Could you check a few things on this drawing? It's one solid part, dimensions in mm from its lowest x, y, z. Give positions to 0.01 mm unless a question says otherwise; leave off trailing zeros. Loops run counter-clockwise (first coordinate to the right, second up) from the corner with the lowest first, then second, coordinate; pieces in that order, holes last. Notation, with made-up numbers: M 32,-20 L 52,-20 A17 ccw 52,-2 Z; hole C 9.25,89 d2. An arc over 180 degrees is marked long. Answer as CSV lines item,"result". Start each with the question number.
Item 1: I want a section at A-A on x = 5. List the corners of the cut face in (y, z) for me, plus the area to 3 significant figures.
Item 2: If we mould it in two halves opening along Y, with no side actions, what happens to the marked faces 1, 2, 3 and 4? For each: released by +Y, released by -Y, zero draft, split by the parting line, or undercut.
Item 3: Will this pin go through, and if not, where does the flat tip stop? P1, Ø2.5, axis at x = 5, y = 5, coming from the -Z side.
Item 4: If I drill on line 1 along X through (y, z) = (5, 2.4); line 2 along Y through (x, z) = (5.75, 4.1), over which ranges is the centre line in solid material (lowest first)? Write a range as from..to.
Item 5: I want a section at B-B on z = 4. List the corners of the cut face in (x, y) for me.
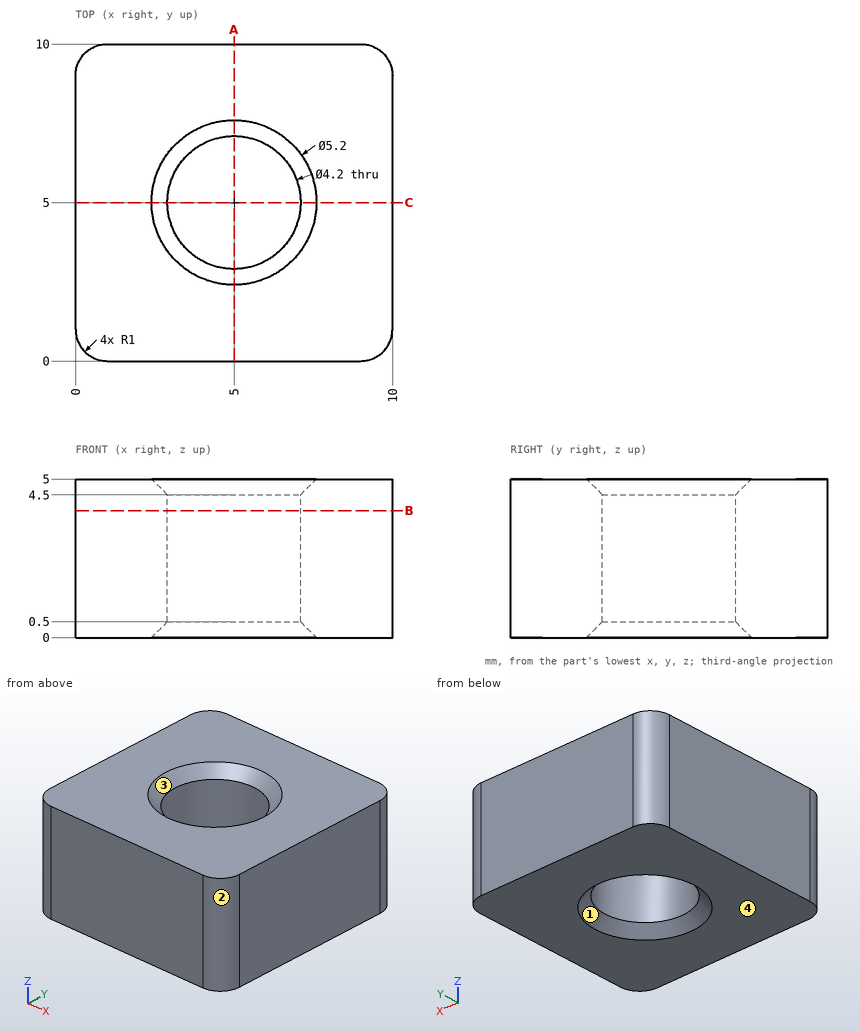
Result:
1,outline,"M 0,0 L 2.4,0 L 2.9,0.5 L 2.9,4.5 L 2.4,5 L 0,5 Z; M 7.1,0.5 L 7.6,0 L 10,0 L 10,5 L 7.6,5 L 7.1,4.5 Z"
1,area,"28.5 mm^2"
2,face 1,"undercut"
2,face 2,"released by -Y"
2,face 3,"undercut"
2,face 4,"zero draft"
3,P1,"through"
4,line 1,"0..2.9, 7.1..10"
4,line 2,"0..3.04, 6.96..10"
5,outline,"M 0,1 A1 ccw 1,0 L 9,0 A1 ccw 10,1 L 10,9 A1 ccw 9,10 L 1,10 A1 ccw 0,9 Z; hole C 5,5 d4.2"
